The drawing under review shows one solid part. Ordinate dimensions are in mm from its lowest x, y, z. Round coordinates to 2 decimals unless told otherwise and drop trailing zeros. Write each loop counter-clockwise with the first axis right and the second up, starting at its lowest first coordinate (ties: lowest second). Pieces come first, ordered by that corner, then holes. Notation, with made-up numbers: (24.25, 36.5) -> (49.25, 36.5) arc R28 cw to (49.25, 73.5) -> close; hole circle Ø9 at (36.5, 12). An arc over 180 degrees is marked (long way). Answer in a Markdown table with one row per item. Add a question column.
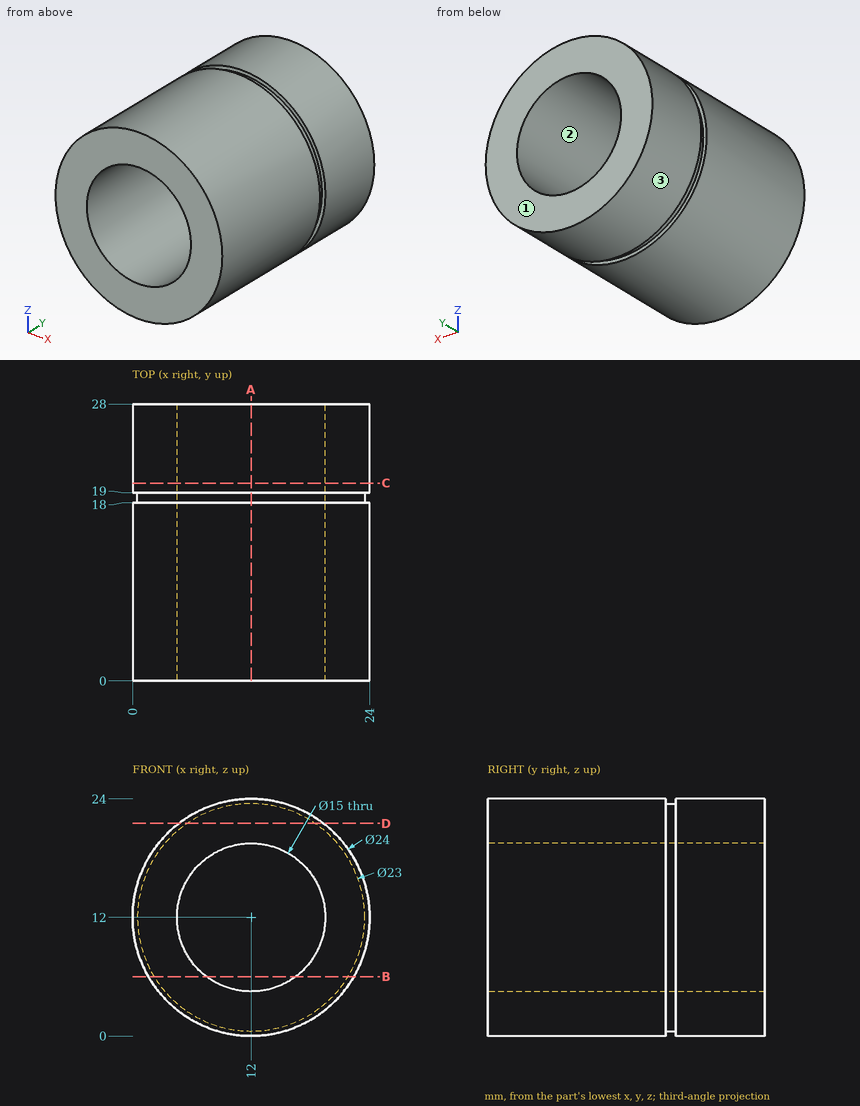
1. Insertion check: pin 1 Ø5 at (x, y) = (15.5, 24) entering from +Z; pin 2 Ø4 at (x, y) = (19, 8.5) entering from +Z; pin 3 Ø1 at (x, y) = (8.5, 11) entering from -Z. Each pin has a flat end and moves straight along its axis. Give the tip position at first contact, or say it passes through.
2. Add section C-C on y = 20. Write out the cut boundary in (x, z).
3. Add section D-D on z = 21.5. Write out the cut boundary in (x, y).
4. For L1, parallel to X at y = 16.5, z = 12; L2, parallel to Z at x = 11, y = 25.75, list the stretches that pass through material, from the lowest coordinate up.
5. Add section A-A on x = 12. Write out the cut boundary in (y, z), plus the area to 3 significant figures.
6. Add section B-B on z = 6. Write out the cut boundary in (x, y).
7. Mouldability with a two-part tool opening along X and no side actions: class the marked faces 1, 2 and 3 as pulls with the +X half, pulls with the -X half, needs draft (parallel to the pull), parting line crosses it, or undercut.
Filled in:
| question | item | result |
|---|---|---|
| 1 | pin 1 | z = 23.96 |
| 1 | pin 2 | z = 22.91 |
| 1 | pin 3 | z = 0.38 |
| 2 | outline | circle Ø24 at (12, 12); hole circle Ø15 at (12, 12) |
| 3 | outline | (4.67, 0) -> (19.33, 0) -> (19.33, 18) -> (18.48, 18) -> (18.48, 19) -> (19.33, 19) -> (19.33, 28) -> (4.67, 28) -> (4.67, 19) -> (5.52, 19) -> (5.52, 18) -> (4.67, 18) -> close |
| 4 | L1 | 0 to 4.5, 19.5 to 24 |
| 4 | L2 | 0.04 to 4.57, 19.43 to 23.96 |
| 5 | outline | (0, 0) -> (18, 0) -> (18, 0.5) -> (19, 0.5) -> (19, 0) -> (28, 0) -> (28, 4.5) -> (0, 4.5) -> close; (0, 19.5) -> (28, 19.5) -> (28, 24) -> (19, 24) -> (19, 23.5) -> (18, 23.5) -> (18, 24) -> (0, 24) -> close |
| 5 | area | 251 mm² |
| 6 | outline | (1.61, 0) -> (7.5, 0) -> (7.5, 28) -> (1.61, 28) -> (1.61, 19) -> (2.19, 19) -> (2.19, 18) -> (1.61, 18) -> close; (16.5, 0) -> (22.39, 0) -> (22.39, 18) -> (21.81, 18) -> (21.81, 19) -> (22.39, 19) -> (22.39, 28) -> (16.5, 28) -> close |
| 7 | face 1 | needs draft |
| 7 | face 2 | undercut |
| 7 | face 3 | parting line crosses it |
